```python
from build123d import *

# Parameters (mm, degrees)
CYLINDER_R             = 1
CYLINDER_DEPTH         = 20
CYLINDER_ROLL_ANGLE    = 90
BOX003_W               = 23
BOX003_H               = 19
BOX003_DEPTH           = 13
BOX004_W               = 33
BOX004_H               = 3
BOX004_DEPTH           = 13
CYLINDER001_R          = 1
CYLINDER001_DEPTH      = 20
CYLINDER001_ROLL_ANGLE = 90
BOX006_W               = 13
BOX006_H               = 6
BOX006_DEPTH           = 10
BOX005_W               = 5
BOX005_H               = 19
BOX005_DEPTH           = 19
CHAMFER_SIZE           = 4
BOX_W                  = 29
BOX_H                  = 6.5
BOX_DEPTH              = 5
BOX001_W               = 4.5
BOX001_H               = 10
BOX001_DEPTH           = 5
BOX002_W               = 40
BOX002_H               = 26
BOX002_DEPTH           = 19


with BuildPart() as cilindro:
    # Cylinder → Cylinder (new body)
    with BuildSketch(Plane.XY):
        Circle(CYLINDER_R)
    extrude(amount=CYLINDER_DEPTH)


with BuildPart() as cilindro_1:
    # Cylinder roll: moved
    add(cilindro.part.rotate(Axis((0, 0, 0), (1, 0, 0)), CYLINDER_ROLL_ANGLE))


with BuildPart() as cilindro_2:
    # Cylinder placement: moved
    add(cilindro_1.part.moved(Location((-2.5, 55, 6.5))))


with BuildPart() as cubo003:
    # Box003 → Box003 (new body)
    with BuildSketch(Plane(origin=(0, 33, 0), x_dir=(1, 0, 0), z_dir=(0, 0, 1))):
        with Locations((11.5, 9.5)):
            Rectangle(BOX003_W, BOX003_H)
    extrude(amount=BOX003_DEPTH)


with BuildPart() as fusion002:
    # Box004 → Box004 (new body)
    with BuildSketch(Plane(origin=(-5, 52, 0), x_dir=(1, 0, 0), z_dir=(0, 0, 1))):
        with Locations((16.5, 1.5)):
            Rectangle(BOX004_W, BOX004_H)
    extrude(amount=BOX004_DEPTH)

    # Fusion002: union Cubo003
    add(cubo003.part)


with BuildPart() as servo_model:
    # Cylinder001 → Cylinder001 (new body)
    with BuildSketch(Plane.XY):
        Circle(CYLINDER001_R)
    extrude(amount=CYLINDER001_DEPTH)


with BuildPart() as servo_model_1:
    # Cylinder001 roll: moved
    add(servo_model.part.rotate(Axis((0, 0, 0), (1, 0, 0)), CYLINDER001_ROLL_ANGLE))


with BuildPart() as servo_model_2:
    # Cylinder001 placement: moved
    add(servo_model_1.part.moved(Location((25.5, 55, 6.5))))

    # Fusion003: union Cilindro, Fusion002
    add(cilindro_2.part)
    add(fusion002.part)


with BuildPart() as servo_model_3:
    # Fusion003 placement: moved
    add(servo_model_2.part.moved(Location((-4, -1, 13))))


with BuildPart() as servo_cable_model:
    # Box006 → Box006 (new body)
    with BuildSketch(Plane(origin=(17, 32, 14.5), x_dir=(1, 0, 0), z_dir=(0, 0, 1))):
        with Locations((6.5, 3)):
            Rectangle(BOX006_W, BOX006_H)
    extrude(amount=BOX006_DEPTH)

    # Fusion005: union Servo_Model
    add(servo_model_3.part)


with BuildPart() as servo_cable_model_1:
    # Fusion005 placement: moved
    add(servo_cable_model.part.moved(Location((0, -28, 0))))


with BuildPart() as chamfer_body:
    # Box005 → Box005 (new body)
    with BuildSketch(Plane(origin=(22, 7, 10), x_dir=(1, 0, 0), z_dir=(0, 0, 1))):
        with Locations((2.5, 9.5)):
            Rectangle(BOX005_W, BOX005_H)
    extrude(amount=BOX005_DEPTH)

    # Chamfer
    chamfer_edges = [chamfer_body.edges().sort_by_distance(p)[0] for p in [
        (27, 7, 19.5),
    ]]
    chamfer(chamfer_edges, length=CHAMFER_SIZE)


with BuildPart() as cubo:
    # Box → Box (new body)
    with BuildSketch(Plane.XY.offset(5)):
        with Locations((14.5, 3.25)):
            Rectangle(BOX_W, BOX_H)
    extrude(amount=BOX_DEPTH)


with BuildPart() as fusion:
    # Box001 → Box001 (new body)
    with BuildSketch(Plane(origin=(5.5, 6.5, 5), x_dir=(1, 0, 0), z_dir=(0, 0, 1))):
        with Locations((2.25, 5)):
            Rectangle(BOX001_W, BOX001_H)
    extrude(amount=BOX001_DEPTH)

    # Fusion: union Cubo
    add(cubo.part)


with BuildPart() as obj1:
    # Box002 → Box002 (new body)
    with BuildSketch(Plane(origin=(-18, 0, 10), x_dir=(1, 0, 0), z_dir=(0, 0, 1))):
        with Locations((20, 13)):
            Rectangle(BOX002_W, BOX002_H)
    extrude(amount=BOX002_DEPTH)

    # Fusion001: union Fusion
    add(fusion.part)

    # Fusion004: union Chamfer body
    add(chamfer_body.part)

    # Cut: cut Servo_Cable_model
    add(servo_cable_model_1.part, mode=Mode.SUBTRACT)


with BuildPart() as obj1_1:
    # Cut placement: moved
    add(obj1.part.moved(Location((0, 0, -5))))


solid = obj1_1.part
```
Can you work these out from the model? Positions are in its coordinate system, mm. A direction names the side the tool comes from. Coordinates: 2 decimals unless noted, no trailing zeros. Loops run counter-clockwise (first coordinate to the right, second up) from the corner with the lowest first, then second, coordinate; pieces in that order, holes last.
Item 1: If we mould it in two halves opening along X, with no side actions, what happens to faces 1 (the face through (-9, 24, 14)), 2 (the face through (22, 3, 14)), 3 (the face through (-7, 6, 15)), 4 (the face through (4, 13, 24))? For each: released by +X, released by -X, zero draft, split by the parting line, or undercut.
Answers below:
face 1: undercut
face 2: released by +X
face 3: undercut
face 4: zero draft
Item 2: I'm going to push flat-ended pins straight in: pin 1 (1.5 mm diameter, centred on y = 12, z = 1.5, fed in from +X); pin 2 (2.5 mm diameter, centred on y = 3.5, z = 2.5, fed in from -X); pin 3 (5 mm diameter, centred on x = 7.5, z = 2, fed in from +Y). Where does each tip first touch, or does it pass through?
Answers below:
pin 1: stops at x = 10
pin 2: stops at x = 0
pin 3: stops at y = 16.5
Item 3: Suppose I cut it at C-C (x = -6.5). Please give me the cut outline in (y, z), then the cut area to 3 significant figures.
Answers below:
outline: (0, 5) - (26, 5) - (26, 8) - (23, 8) - (23, 13.5) - (6, 13.5) - (6, 15.5) - (23, 15.5) - (23, 21) - (26, 21) - (26, 24) - (0, 24) - close
area: 421 mm2
Item 4: Suppose I cut it at D-D (x = 20). Please give me the cut outline in (y, z), then the cut area to 4 significant figures.
Answers below:
outline: (0, 0) - (6.5, 0) - (6.5, 5) - (26, 5) - (26, 8) - (23, 8) - (23, 21) - (26, 21) - (26, 24) - (0, 24) - close; hole (4, 9.5) - (10, 9.5) - (10, 19.5) - (4, 19.5) - close
area: 427.5 mm2
Item 5: Please list where these lines run through material, in increasing order: L1, parallel to X at y = 15.75, z = 14.5; L2, parallel to Z at x = 12.5, y = 8.25; L3, parallel to Y at x = 20.5, z = 9.75.
Answers below:
L1: x = -18 to -7.5, -5.5 to -4, 19 to 20.5, 22.5 to 27
L2: z = 5 to 8, 21 to 24
L3: y = 0 to 4, 10 to 23
Item 6: Which directions (+Z, -Z, +X, -X, +Y, -Y) give clear straight access to the entire face, cutting with the end or side of a thin tool? Please do faces 5 (the face through (22, 8, 19.5)), 6 (the face through (5.5, 11, 2)), 7 (the face through (-4, 13, 14)), 8 (the face through (22.5, 7, 7.2)).
Answers below:
face 5: +X
face 6: -Z, -X, +Y
face 7: +Y
face 8: +Z, -Z, +X, -Y
Item 7: Suppose I cut it at B-B (y = 8.5). Please give me the cut outline in (x, z), then the cut area to 3 significant figures.
Answers below:
outline: (-18, 5) - (5.5, 5) - (5.5, 0) - (10, 0) - (10, 5) - (24.5, 5) - (24.5, 9.5) - (19, 9.5) - (19, 8) - (-4, 8) - (-4, 21) - (19, 21) - (19, 19.5) - (24.5, 19.5) - (24.5, 24) - (-18, 24) - close; hole circle Ø2 at (-6.5, 14.5)
area: 473 mm2
Item 8: Suppose I cut it at A-A (z = 14.5). Please give me the cut outline in (x, y), then the cut area to 4 significant figures.
Answers below:
outline: (-18, 0) - (22, 0) - (22, 4) - (-4, 4) - (-4, 23) - (-5.5, 23) - (-5.5, 6) - (-7.5, 6) - (-7.5, 23) - (-9, 23) - (-9, 26) - (-18, 26) - close; (19, 10) - (20.5, 10) - (20.5, 23) - (19, 23) - close; (22.5, 10) - (26, 10) - (27, 11) - (27, 26) - (24, 26) - (24, 23) - (22.5, 23) - close
area: 505.5 mm2
